Design review of the part built by this model. Coordinates are the model's own, in mm. A direction names the side the tool comes from. Give positions to 0.01 mm unless a question says otherwise; leave off trailing zeros. Write each loop counter-clockwise with the first axis right and the second up, starting at its lowest first coordinate (ties: lowest second). Pieces come first, ordered by that corner, then holes.
```python
from build123d import *

# Parameters (mm, degrees)
BOSS_EXTRU_1_DEPTH = 5


with BuildPart() as part:
    # Esquisse1 → Boss.-Extru.1 (new body)
    with BuildSketch(Plane.XY):
        Polygon((-41.749094475, 67.928932188), (-48.820162287, 75), (-48.820162287, 0), (-43.820162287, 0), (-43.820162287, -5), (-33.820162287, -5), (-33.820162287, 0), (-10, 0), (-10, -5), (0, -5), (0, 0), (0, 26.179837713), (-13.535533906, 39.715371619), (-24.142135624, 50.321973337), (-34.678026663, 60.857864376), align=None)
        Polygon((-43.820162287, 75), (-48.820162287, 75), (-41.749094475, 67.928932188), (-38.213560569, 71.464466094), (-31.142492757, 64.393398282), (-34.678026663, 60.857864376), (-24.142135624, 50.321973337), (-20.606601718, 53.857507243), (-10, 43.250905525), (-13.535533906, 39.715371619), (0, 26.179837713), (0, 75), (0, 80), (-10, 80), (-10, 75), (-33.820162287, 75), (-33.820162287, 80), (-43.820162287, 80), align=None)
    extrude(amount=BOSS_EXTRU_1_DEPTH)


solid = part.part
```
(1) Mouldability with a two-part tool opening along Y and no side actions: class faces 6 (the face through (-22, 75, 2)), 7 (the face through (-22.399, 52.065, 2.465)), 8 (the face through (-46, 0, 2)) as pulls with the +Y half, pulls with the -Y half, needs draft (parallel to the pull), parting line crosses it, or undercut.
Resolved:
face 6: pulls with the +Y half
face 7: undercut
face 8: pulls with the -Y half
(2) To check wall thickness, follow L1, parallel to X at y = 77.5, z = 2.3; L2, parallel to Y at x = -37, z = 1.25; L3, parallel to X at y = 44.5, z = 1.6. State the ranges of each line that lie inside material, in increasing order.
Resolved:
L1: x = -43.82 to -33.82, -10 to 0
L2: y = -5 to 63.18, 70.25 to 80
L3: x = -48.82 to -18.32, -11.25 to 0
(3) Consider section A-A, the plane x = -22.5. Give the boundary of the cut face in (y, z).
Resolved:
outline: (0, 0) - (48.68, 0) - (48.68, 5) - (0, 5) - close; (51.96, 0) - (75, 0) - (75, 5) - (51.96, 5) - close
(4) Tool access review of faces 1 (the face through (-46, 75, 2)), 2 (the face through (-5, -5, 2)), 3 (the face through (-43.82, -2, 2)), 4 (the face through (-40.01, 69.67, 2.46)), 5 (the face through (-33.82, -3, 2)): name each direction out of +Z, -Z, +X, -X, +Y, -Y from which nothing blocks a thin tool from reaching the whole face with its end or side.
Resolved:
face 1: +Z, -Z, -X, +Y
face 2: +Z, -Z, +X, -X, -Y
face 3: +Z, -Z, -X, -Y
face 4: +Z, -Z
face 5: +Z, -Z, -Y
(5) Clearance check with flat-ended pins moving along their axes: P1, Ø1.5, axis at y = 78.5, z = 2.5, coming from the -X side; P2, Ø1.5, axis at x = -45.5, z = 3.5, coming from the -Y side; P3, Ø2.5, axis at x = -46.5, z = 3.5, coming from the +Y side. State where each tip first meets the part, or that it passes through.
Resolved:
P1: stops at x = -43.82
P2: stops at y = 0
P3: stops at y = 75
(6) Consider section B-B, the plane z = 0.8. Give the boundary of the cut face in (x, y), then the cut area to 3 significant figures.
Resolved:
outline: (-48.82, 0) - (-43.82, 0) - (-43.82, -5) - (-33.82, -5) - (-33.82, 0) - (-10, 0) - (-10, -5) - (0, -5) - (0, 80) - (-10, 80) - (-10, 75) - (-33.82, 75) - (-33.82, 80) - (-43.82, 80) - (-43.82, 75) - (-48.82, 75) - close; hole (-41.75, 67.93) - (-34.68, 60.86) - (-31.14, 64.39) - (-38.21, 71.46) - close; hole (-24.14, 50.32) - (-13.54, 39.72) - (-10, 43.25) - (-20.61, 53.86) - close
area: 3,740 mm2
(7) Consider section C-C, the plane x = -17.5. Give the boundary of the cut face in (y, z), then the cut area to 3 significant figures.
Resolved:
outline: (0, 0) - (43.68, 0) - (43.68, 5) - (0, 5) - close; (50.75, 0) - (75, 0) - (75, 5) - (50.75, 5) - close
area: 340 mm2
